Autodesk Inventor part; units mm, degrees
ref_plane "YZ Plane" through (0, 0, 0) normal (1, 0, 0) x (0, 1, 0)
ref_plane "XZ Plane" through (0, 0, 0) normal (0, 1, 0) x (-1, 0, 0)
ref_plane "XY Plane" through (0, 0, 0) normal (0, 0, 1) x (1, 0, 0)
sketch "Sketch1" plane through (0, 0, 0) normal (0, 0, 1) x (1, 0, 0)
  line L0 (-2.05, 2.05) -> (2.05, 2.05)
  line L1 (2.05, 2.05) -> (2.05, -2.05)
  line L2 (2.05, -2.05) -> (-2.05, -2.05)
  line L3 (-2.05, -2.05) -> (-2.05, 2.05)
  line L4 (0, 2.05) -> (0, -2.05) construction
  line L5 (0, 7.5) -> (-15.55, 7.5)
  line L6 (-15.55, 7.5) -> (-15.55, 6)
  line L7 (-15.55, 6) -> (-3.55, 6)
  line L8 (-3.55, 6) -> (-3.55, -6)
  line L9 (-3.55, -6) -> (-15.55, -6)
  line L10 (-15.55, -6) -> (-15.55, -7.5)
  line L11 (-15.55, -7.5) -> (-0.55, -7.5)
  line L12 (-2.05, 0) -> (2.05, 0) construction
  line L13 (0, 7.5) -> (15.55, 7.5)
  line L14 (15.55, 7.5) -> (15.55, 6)
  line L15 (15.55, 6) -> (3.55, 6)
  line L16 (3.55, 6) -> (3.55, -6)
  line L17 (3.55, -6) -> (15.55, -6)
  line L18 (15.55, -6) -> (15.55, -7.5)
  line L19 (15.55, -7.5) -> (-0.55, -7.5)
  line L20 (-2.05, 2.05) -> (2.05, -2.05) construction
  line L21 (2.05, 2.05) -> (-2.05, -2.05) construction
  line L22 (0, 7.5) -> (0, 2.05) construction
  line L23 (-3.55, 6) -> (-3.55, 7.5)
  line L24 (-3.55, -6) -> (-3.55, -7.5)
  line L25 (3.55, 6) -> (3.55, 7.5)
  line L26 (3.55, -6) -> (3.55, -7.5)
  point P0 (0, 0)
  point P1 (0, 0)
  point P2 (0, 0)
  dimension "d3" = 4.1
  dimension "d4" = 4.1
  dimension "d5" = 12
  dimension "d6" = 1.5
  dimension "d7" = 1.5
  dimension "d8" = 5.45
  dimension "d9" = 5.45
  dimension "d10" = 1.5
  dimension "d11" = 12
  dimension "d37" = 15
extrude "Extrusion1" add sketch "Sketch1" along normal blind 10 contours L13 L25 L16 L26 L19 L11 L24 L8 L23 L5
sketch "Sketch5" plane through (0, 0, 10) normal (0, 0, 1) x (1, 0, 0)
  line L0 (6, 19.5) -> (7.5, 19.5)
  line L1 (7.5, 19.5) -> (7.5, 7.5)
  line L2 (7.5, 7.5) -> (6, 7.5)
  line L3 (6, 7.5) -> (6, 19.5)
  line L4 (3.55, 7.5) -> (-3.55, 7.5)
  line L5 (3.55, -7.5) -> (3.55, 7.5)
  line L6 (0, 0) -> (0, 23.4065) construction
  point P0 (15.55, 7.5)
  point P1 (-15.55, 7.5)
  point P2 (3.55, -6)
  point P3 (3.55, 6)
  dimension "d41" = 1.5
  dimension "d42" = 12
  dimension "d47" = 6
extrude "Extrusion5" add sketch "Sketch5" against normal up to surface (10 mm away)
mirror "Mirror1" about plane through (0, 0, 0) normal (1, 0, 0) of "Extrusion5"
sketch "Sketch7" plane through (0, 0, 10) normal (0, 0, 1) x (1, 0, 0)
  line L0 (-7.5, 19.5) -> (-7.5, 7.5)
  line L1 (-7.5, 7.5) -> (7.5, 7.5)
  line L2 (7.5, 7.5) -> (7.5, 6)
  line L3 (7.5, 6) -> (-7.5, 6)
  line L4 (-7.5, 6) -> (-7.5, 7.5)
  line L5 (7.5, 7.5) -> (7.5, 19.5)
  point P0 (0, 0)
  dimension "d53" = 1.5
extrude "Extrusion7" add sketch "Sketch7" against normal up to surface (10 mm away)
fillet "Fillet3" radius 1 4 edges at (-3.55, 6, 5) (3.55, 6, 5) (7.5, 6, 5) (-7.5, 6, 5)
sketch "Sketch8" plane through (0, 0, 10) normal (0, 0, 1) x (1, 0, 0)
  line L0 (-3.55, -3.55) -> (3.55, -3.55)
  line L1 (3.55, -3.55) -> (3.55, -7.5)
  line L2 (3.55, -7.5) -> (-3.55, -7.5)
  line L3 (-3.55, -7.5) -> (-3.55, -3.55)
  line L4 (2.05, -2.05) -> (-2.05, -2.05)
  line L5 (3.55, -7.5) -> (3.55, 5)
  line L6 (-3.55, 5) -> (-3.55, -7.5)
  line L7 (-3.55, -7.5) -> (3.55, -7.5)
  point P0 (0, 0)
  dimension "d57" = 1.5
extrude "Extrusion8" cut sketch "Sketch8" against normal blind 10
equation "\"d7\" = d6"
equation "\"d8\" = d9"
properties part number "Rudder_interface" material "ABS Plastic"
Check sheet for the modelled part. Datum: model origin and axes. Units: mm. A direction names the side the tool comes from. Give positions to 0.01 mm unless a question says otherwise; leave off trailing zeros. Write each loop counter-clockwise with the first axis right and the second up, starting at its lowest first coordinate (ties: lowest second). Pieces come first, ordered by that corner, then holes. Notation, with made-up numbers: (-30, -6) -> (25, -6) arc R28 ccw to (25, 13) -> close; hole circle Ø11 at (66.5, -16). An arc over 180 degrees is marked (long way). Write item = value, one per line.
Item 1: Scan lines: probe 1 along X at (y, z) = (16.25, 3.75); probe 2 along X at (y, z) = (-1, 3.75); probe 3 along Y at (x, z) = (-0.5, 2.75). Record each from-to range of solid material in increasing order. Write a range as from..to.
Output:
probe_1 = -7.5..-6, 6..7.5
probe_2 = -3.55..-2.05, 2.05..3.55
probe_3 = -3.55..-2.05, 2.05..7.5
Item 2: Release check for a two-part mould opening along X. For faces 5 (the flat face through (7, 19.5, 5)), 6 (the flat face through (7.5, 13, 5)), 7 (the flat face through (2.05, 0, 5)), 8 (the flat face through (0, -2.05, 5)) record: +X half, -X half, draft (parallel to the pull), parting line (faces both ways), or undercut.
Output:
face_5 = draft
face_6 = +X half
face_7 = undercut
face_8 = undercut
Item 3: Sectioned sample at D-D on x = 3.25. Record the boundary of the cut face in (y, z).
Output:
outline = (-3.55, 0) -> (7.5, 0) -> (7.5, 10) -> (-3.55, 10) -> close
Item 4: Sectioned sample at C-C on y = -1. Record the boundary of the cut face in (x, z), and give its area (3 significant figures).
Output:
outline = (-3.55, 0) -> (-2.05, 0) -> (-2.05, 10) -> (-3.55, 10) -> close; (2.05, 0) -> (3.55, 0) -> (3.55, 10) -> (2.05, 10) -> close
area = 30.0 mm^2
Item 5: Sectioned sample at B-B on z = 8.5. Record the boundary of the cut face in (x, y).
Output:
outline = (-7.5, 7) arc R1 ccw to (-6.5, 6) -> (-4.55, 6) arc R1 cw to (-3.55, 5) -> (-3.55, -3.55) -> (3.55, -3.55) -> (3.55, 5) arc R1 cw to (4.55, 6) -> (6.5, 6) arc R1 ccw to (7.5, 7) -> (7.5, 19.5) -> (6, 19.5) -> (6, 7.5) -> (-6, 7.5) -> (-6, 19.5) -> (-7.5, 19.5) -> close; hole (-2.05, -2.05) -> (2.05, -2.05) -> (2.05, 2.05) -> (-2.05, 2.05) -> close
Item 6: Tool access check on faces 1 (the flat face through (6, 6, 5)), 2 (the flat face through (0, 7.5, 5)), 3 (the flat face through (-3.55, 1, 5)), 4 (the flat face through (0, 2.05, 5)). Record the directions out of +Z, -Z, +X, -X, +Y, -Y that give a thin tool (end or side, any length) a straight path to the whole face; none if there is none.
Output:
face_1 = +Z, -Z, +X, -Y
face_2 = +Z, -Z, +Y
face_3 = +Z, -Z, -X, -Y
face_4 = +Z, -Z
Item 7: Sectioned sample at A-A on x = 0.5. Record the boundary of the cut face in (y, z), and give its area (3 significant figures).
Output:
outline = (-3.55, 0) -> (-2.05, 0) -> (-2.05, 10) -> (-3.55, 10) -> close; (2.05, 0) -> (7.5, 0) -> (7.5, 10) -> (2.05, 10) -> close
area = 69.5 mm^2
Item 8: Gauge pin test, flat ends, axial feed: pin 1 (4.5 mm diameter, centred on y = 1, z = 6, fed in from -X); pin 2 (6 mm diameter, centred on x = -1.5, y = 15.5, fed in from -Z); pin 3 (4.5 mm diameter, centred on y = -1, z = 6.5, fed in from +X); pin 4 (2 mm diameter, centred on x = 0, z = 2.5, fed in from +Y). Record the tip position at first contact, or that the pin passes through.
Output:
pin_1 = -3.55
pin_2 = through
pin_3 = 3.55
pin_4 = 7.5
